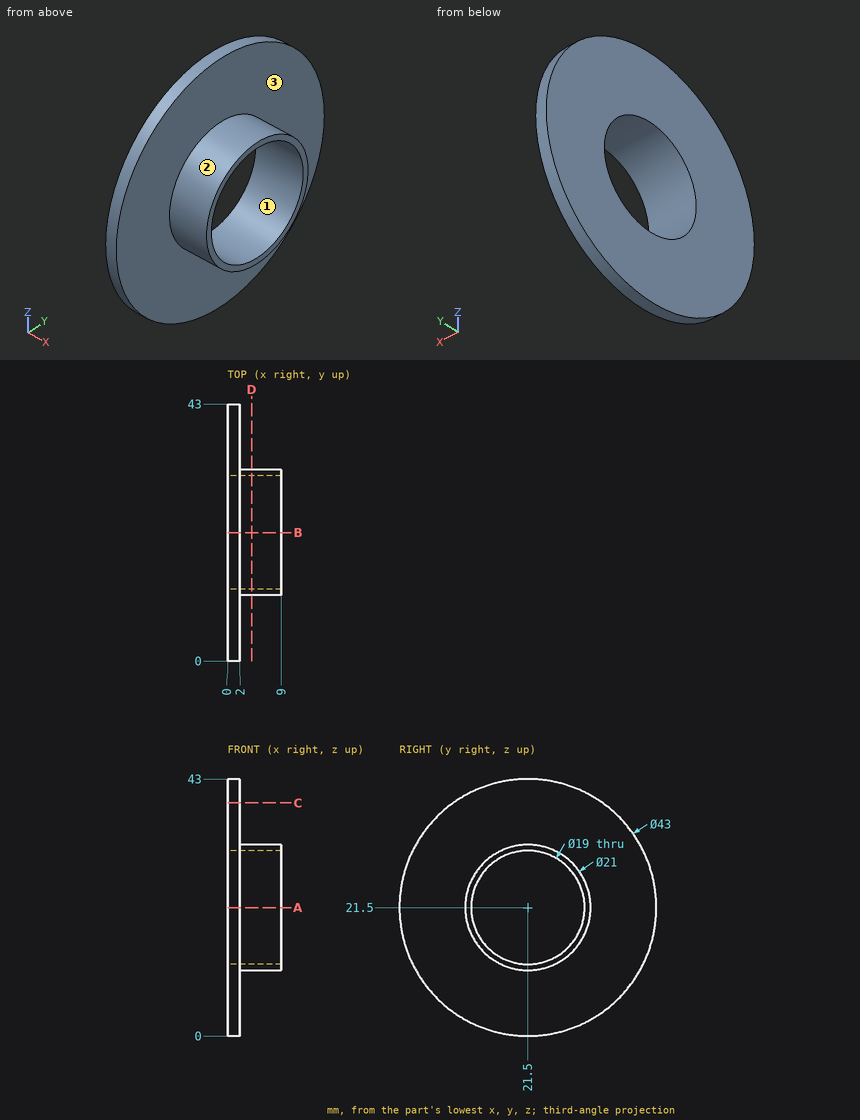
Geometry check sheet. Reference: drawing and pictorial views, mm from the part's lowest x, y, z. Round coordinates to 2 decimals unless told otherwise and drop trailing zeros. Loops run counter-clockwise (first coordinate to the right, second up) from the corner with the lowest first, then second, coordinate; pieces in that order, holes last. Notation, with made-up numbers: (45.25, 70) -> (75.25, 70) arc R24 cw to (75.25, 95) -> close; hole circle Ø5 at (62.25, -35). An arc over 180 degrees is marked (long way). Use a Markdown table: item, result.
(1) Mould release check, pull along Y, two halves, no side actions. Record for the marked faces 1, 2 and 3: released by +Y, released by -Y, zero draft, split by the parting line, or undercut.
Calculated:
| item | result |
|---|---|
| face 1 | undercut |
| face 2 | split by the parting line |
| face 3 | zero draft |
(2) Go/stop test with flat-tipped pins: P1, Ø12, axis at y = 27.5, z = 27.5, coming from the +X side; P2, Ø1.5, axis at y = 8, z = 27.5, coming from the +X side; P3, Ø1.5, axis at x = 6, z = 21.5, coming from the +Y side; P4, Ø1, axis at x = 2, z = 24.5, coming from the -Y side. Record where each tip stops, or that it passes through.
Calculated:
| item | result |
|---|---|
| P1 | x = 9 |
| P2 | x = 2 |
| P3 | y = 32 |
| P4 | y = 0.15 |
(3) Sectioned sample at A-A (z = 21.5). Enter the section's corners in (x, y), then the cut area to 3 significant figures.
Calculated:
| item | result |
|---|---|
| outline | (0, 0) -> (2, 0) -> (2, 11) -> (9, 11) -> (9, 12) -> (0, 12) -> close; (0, 31) -> (9, 31) -> (9, 32) -> (2, 32) -> (2, 43) -> (0, 43) -> close |
| area | 62.0 mm² |
(4) Sectioned sample at C-C (z = 39). Enter the section's corners in (x, y).
Calculated:
| item | result |
|---|---|
| outline | (0, 9.01) -> (2, 9.01) -> (2, 33.99) -> (0, 33.99) -> close |
(5) Scan lines: probe 1 along Y at (x, z) = (3.5, 21.5); probe 2 along X at (y, z) = (38, 29); probe 3 along Y at (x, z) = (7.75, 19). Record each from-to range of solid material in increasing order.
Calculated:
| item | result |
|---|---|
| probe 1 | 11 to 12, 31 to 32 |
| probe 2 | 0 to 2 |
| probe 3 | 11.3 to 12.33, 30.67 to 31.7 |
(6) Sectioned sample at D-D (x = 4). Enter the section's corners in (y, z).
Calculated:
| item | result |
|---|---|
| outline | circle Ø21 at (21.5, 21.5); hole circle Ø19 at (21.5, 21.5) |
